Input: part model. Units: mm. Frame: model coordinates. A direction names the side the tool comes from. Coordinates: 2 decimals unless noted, no trailing zeros. Order: outer loops, then holes, each group sorted by start corner. A loop starts at its lowest first (then second) coordinate and runs counter-clockwise, first axis right, second up. Notation, with made-up numbers: (-33.75, -35) -> (10.25, -35) arc R27 ccw to (10.25, 4) -> close; hole circle Ø9 at (13, 29.25). An arc over 180 degrees is marked (long way). One line per question, with ' | ' between items.
```python
from build123d import *

# Parameters (mm, degrees)
CUT_EXTRUDE1_DEPTH = 6.35
CHAMFER1_SIZE      = 0.9652
CHAMFER2_SIZE      = 0.9652


with BuildPart() as part:
    # Sketch1 → Revolve1 (revolve)
    with BuildSketch(Plane(origin=(0, 0, 0), x_dir=(1, 0, 0), z_dir=(0, 1, 0))):
        Polygon((0, 52.830247514), (0, 11.555247514), (-4.7625, 11.555247514), (-4.7625, 40.917647514), (-8.6741, 40.917647514), (-8.6741, 43.305247514), (-7.14375, 43.305247514), (-7.14375, 52.830247514), align=None)
    revolve(axis=Axis((0, 0, -86.603340611), (0, 0, 1)))

    # Sketch2 → Cut-Extrude1 (cut)
    with BuildSketch(Plane(origin=(0, 0, -52.830247514), x_dir=(-1, 0, 0), z_dir=(0, 0, -1))):
        Polygon((2.27302801, 3.937), (-2.27302801, 3.937), (-4.54605602, 0), (-2.27302801, -3.937), (2.27302801, -3.937), (4.54605602, 0), align=None)
    extrude(amount=-CUT_EXTRUDE1_DEPTH, mode=Mode.SUBTRACT)

    # Chamfer1
    chamfer1_edges = [part.edges().sort_by_distance(p)[0] for p in [
        (4.7625, 0, -11.555247514),
    ]]
    chamfer(chamfer1_edges, length=CHAMFER1_SIZE)

    # Chamfer2
    chamfer2_edges = [part.edges().sort_by_distance(p)[0] for p in [
        (7.14375, 0, -52.830247514),
    ]]
    chamfer(chamfer2_edges, length=CHAMFER2_SIZE)


solid = part.part
```
1. Cut plane B-B, the plane z = -17. Return loops of the section in (x, y) (1 decimal), and give its area (3 significant figures).
Recorded:
outline: circle Ø9.5 at (0, 0) | area: 71.3 mm^2
2. Pin query (flat end, axial travel): pin 1 Ø1.5 at (x, z) = (-3, -22) entering from -Y; pin 2 Ø2.5 at (x, y) = (-0.5, -1.5) entering from -Z; pin 3 Ø5 at (x, z) = (-5, -48.5) entering from +Y. Return the tip coordinate at first contact, or that it passes through.
Recorded:
pin 1: stops at y = -4.2 | pin 2: stops at z = -46.48 | pin 3: stops at y = 6.69
3. Ray query, line 1 (Z direction, x = 0.75, y = 7.25); line 2 (Z direction, x = -1, y = 1); line 3 (Y direction, x = 4.5, z = -49.5). Return the intervals inside material, ascending. Write a range as [from, to].
Recorded:
line 1: z = [-43.31, -40.92] | line 2: z = [-46.48, -11.56] | line 3: y = [-5.55, -0.08], [0.08, 5.55]
4. Mould query, pull axis Y, two halves, no side actions, for faces 4 (the face through (-4, 1.3, -52.83)), 5 (the face through (0, 0, -46.48)), 6 (the face through (1.88, 8.468, -42.128)). Classes: released by +Y, released by -Y, zero draft, split by the parting line, or undercut.
Recorded:
face 4: zero draft | face 5: undercut | face 6: split by the parting line
5. Access query for faces 1 (the face through (0, 0, -11.555)), 2 (the face through (-3.425, 1.941, -49.7)), 3 (the face through (4, 4, -40.918)). Directions: +Z, -Z, +X, -X, +Y, -Y. A direction counts if a zero-diameter tool reaches every point of the face in a straight line with its end or side. Return the directions, or none.
Recorded:
face 1: +Z, +X, -X, +Y, -Y | face 2: -Z | face 3: +Z
6. Cut plane A-A, the plane x = 0. Return loops of the section in (y, z).
Recorded:
outline: (-8.67, -43.31) -> (-7.14, -43.31) -> (-7.14, -51.87) -> (-6.18, -52.83) -> (-3.94, -52.83) -> (-3.94, -46.48) -> (3.94, -46.48) -> (3.94, -52.83) -> (6.18, -52.83) -> (7.14, -51.87) -> (7.14, -43.31) -> (8.67, -43.31) -> (8.67, -40.92) -> (4.76, -40.92) -> (4.76, -12.52) -> (3.8, -11.56) -> (-3.8, -11.56) -> (-4.76, -12.52) -> (-4.76, -40.92) -> (-8.67, -40.92) -> close
